Geometry: final body of the model. Coordinates: model frame, mm. A direction names the side the tool comes from. Round coordinates to 2 decimals unless told otherwise and drop trailing zeros. Order: outer loops, then holes, each group sorted by start corner. A loop starts at its lowest first (then second) coordinate and runs counter-clockwise, first axis right, second up. Notation, with made-up numbers: (41, 58.25) - (49, 58.25) arc R26 cw to (49, 97.25) - close; hole circle Ø6 at (22.5, -37.5). An arc over 180 degrees is marked (long way). Put each result on its own line as item: value. Start each with the question number.
(1) Access query for faces 1 (the face through (0, 13, 0)), 2 (the face through (-3.937, 940, 0)), 3 (the face through (-7.112, 940, 0)). Directions: +Z, -Z, +X, -X, +Y, -Y. A direction counts if a zero-diameter tool reaches every point of the face in a straight line with its end or side. Return the directions, or none.
(2) Section A-A (y = 531). Output: boundary loops of the cut face in (x, z).
(3) Material intervals for L1, parallel to X at y = 263, z = 1.75; L2, parallel to X at y = 729.5, z = 8.5, sorted ascending. Write a range as [from, to].
(4) Pin query (flat end, axial travel): P1, Ø1, axis at y = 114, z = 7, coming from the +X side; P2, Ø7.5, axis at y = 942.848, z = 0, coming from the +X side; P3, Ø5, axis at y = 776, z = -2.5, coming from the +X side; P4, Ø4.5, axis at y = 9.652, z = 0, coming from the +X side. Return the tip coordinate at first contact, or that it passes through.
from build123d import *

# Parameters (mm, degrees)
BOSS_EXTRUDE1_DEPTH     = 12.7
FILLET1_R               = 7.62
CUT_EXTRUDE1_DEPTH      = 953.611211641
CUT_EXTRUDE1_DEPTH_BACK = 953.611211641
SKETCH2_R               = 2.413


with BuildPart() as part:
    # Sketch1 → Boss-Extrude1 (new, symmetric)
    with BuildSketch(Plane.XY):
        Polygon((0, 0), (3.175, 0), (3.175, 25.4), (-3.937, 927.1), (-3.937, 952.5), (-7.112, 952.5), (-7.112, 927.1), (0, 25.4), align=None)
    extrude(amount=BOSS_EXTRUDE1_DEPTH, both=True)

    # Fillet1
    fillet1_edges = [part.edges().sort_by_distance(p)[0] for p in [
        (1.5875, 0, -12.7),
        (-5.5245, 952.5, 12.7),
        (1.5875, 0, 12.7),
        (-5.5245, 952.5, -12.7),
    ]]
    fillet(fillet1_edges, radius=FILLET1_R)

    # Sketch2 → Cut-Extrude1 (cut, two sides: drawn at the far end of the back side and taken through both)
    with BuildSketch(Plane(origin=(-3.937, 0, 0), x_dir=(0, 0, -1), z_dir=(1, 0, 0)).offset(-CUT_EXTRUDE1_DEPTH_BACK)):
        with Locations((0, 942.848)):
            Circle(SKETCH2_R)
        with Locations((0, 9.652)):
            Circle(SKETCH2_R)
    extrude(amount=CUT_EXTRUDE1_DEPTH + CUT_EXTRUDE1_DEPTH_BACK, mode=Mode.SUBTRACT)


solid = part.part
Checks:
1. face 1: +Z, -Z, -X, -Y
1. face 2: +Z, -Z, +X, +Y
1. face 3: +Z, -Z, -X, +Y, -Y
2. outline: (-3.99, -12.7) - (-0.81, -12.7) - (-0.81, 12.7) - (-3.99, 12.7) - close
3. L1: x = [-1.87, 1.3]
3. L2: x = [-5.55, -2.38]
4. P1: stops at x = 2.48
4. P2: stops at x = -3.94
4. P3: stops at x = -2.73
4. P4: passes through
